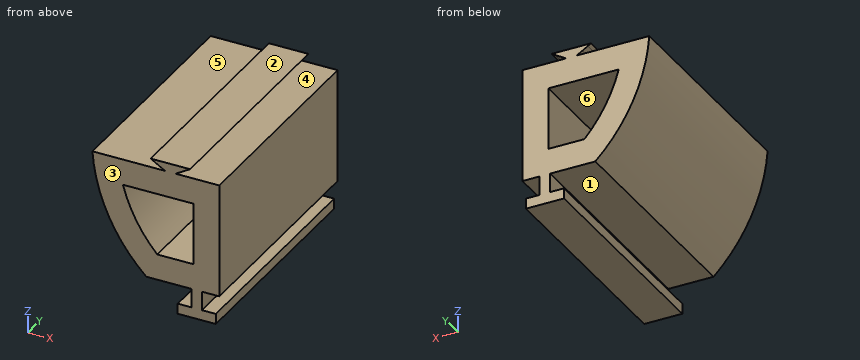
```python
from build123d import *

# Parameters (mm, degrees)
SKETCH1_W           = 0.6
SKETCH1_H           = 0.2
BOSS_EXTRUDE1_DEPTH = 13
CUT_EXTRUDE1_DEPTH  = 14


with BuildPart() as part:
    # Sketch1 → Boss-Extrude1 (new body)
    with BuildSketch(Plane(origin=(0, 0, 0), x_dir=(1, 0, 0), z_dir=(0, 1, 0))):
        with BuildLine():
            Line((-2.7, 0.7), (-2.7, 7.3))
            Line((-2.7, 7.3), (-3.7, 7.3))
            Line((-3.7, 7.3), (-4.3, 7.3))
            Line((-4.3, 7.3), (-6.907423543, 7.3))
            ThreePointArc((-6.907423543, 7.3), (-9.08690024, 4.293104241), (-10.025592252, 0.7))
            Line((-10.025592252, 0.7), (-6.025, 0.7))
            Line((-6.025, 0.7), (-5.830634937, 0.7))
            Line((-5.830634937, 0.7), (-5.219365063, 0.7))
            Line((-5.219365063, 0.7), (-5.025, 0.7))
            Line((-5.025, 0.7), (-2.7, 0.7))
        make_face()
        Polygon((-5.076449576, 0.614250707), (-5.219365063, 0.7), (-5.830634937, 0.7), (-5.973550424, 0.614250707), (-6.16396827, 0.5), (-4.88603173, 0.5), align=None)
        Polygon((-4.576449576, 0.314250707), (-4.88603173, 0.5), (-6.16396827, 0.5), (-6.473550424, 0.314250707), (-6.66396827, 0.2), (-4.38603173, 0.2), align=None)
        with Locations((-4, 7.4)):
            Rectangle(SKETCH1_W, SKETCH1_H)
        with BuildLine():
            Line((-4.3, 7.5), (-3.7, 7.5))
            Line((-3.7, 7.5), (-3.7, 8.4))
            Line((-3.7, 8.4), (-2.9, 8.4))
            Line((-2.9, 8.4), (-2.9, 9))
            Line((-2.9, 9), (-4.472415455, 9))
            ThreePointArc((-4.472415455, 9), (-4.789229045, 8.835484432), (-5.1, 8.659821014))
            Line((-5.1, 8.659821014), (-5.1, 8.4))
            Line((-5.1, 8.4), (-4.3, 8.4))
            Line((-4.3, 8.4), (-4.3, 7.5))
        make_face()
        with BuildLine():
            Line((-5.1, 8.891147283), (-5.1, 8.659821014))
            ThreePointArc((-5.1, 8.659821014), (-4.789229045, 8.835484432), (-4.472415455, 9))
            Line((-4.472415455, 9), (-4.905354218, 9))
            ThreePointArc((-4.905354218, 9), (-5.002973164, 8.946103035), (-5.1, 8.891147283))
        make_face()
        with BuildLine():
            Line((-5.1, 9), (-5.1, 8.891147283))
            ThreePointArc((-5.1, 8.891147283), (-5.002973164, 8.946103035), (-4.905354218, 9))
            Line((-4.905354218, 9), (-5.1, 9))
        make_face()
    extrude(amount=BOSS_EXTRUDE1_DEPTH)

    # Sketch2 → Cut-Extrude1 (cut, through all)
    with BuildSketch(Plane(origin=(0, 13, 0), x_dir=(1, 0, 0), z_dir=(0, 1, 0))):
        with BuildLine():
            Line((-4.2, 5.8), (-6.281918497, 5.8))
            ThreePointArc((-6.281918497, 5.8), (-7.491475696, 4.120714974), (-8.262112321, 2.2))
            Line((-8.262112321, 2.2), (-4.2, 2.2))
            Line((-4.2, 2.2), (-4.2, 5.8))
        make_face()
    extrude(amount=-CUT_EXTRUDE1_DEPTH, mode=Mode.SUBTRACT)


solid = part.part
```
The model under review builds one solid part; all positions refer to its coordinate system, in mm. Face numbers are marked on the shaded views. A direction names the side the tool comes from. Round coordinates to 2 decimals unless told otherwise and drop trailing zeros. Loops run counter-clockwise (first coordinate to the right, second up) from the corner with the lowest first, then second, coordinate; pieces in that order, holes last. Notation, with made-up numbers: (-34.5, 71) -> (15.5, 71) arc R23 cw to (15.5, 88) -> close; hole circle Ø2 at (83, 80). An arc over 180 degrees is marked (long way). Answer in a Markdown table with one row per item.
1) Tool access review of the marked faces 4, 5 and 6: name each direction out of +Z, -Z, +X, -X, +Y, -Y from which nothing blocks a thin tool from reaching the whole face with its end or side.
Taken from the geometry:
| item | result |
|---|---|
| face 4 | +X, +Y, -Y |
| face 5 | -X, +Y, -Y |
| face 6 | +Y, -Y |
2) Consider section A-A, the plane x = -5.5. Write out the cut boundary in (y, z).
Taken from the geometry:
| item | result |
|---|---|
| outline | (0, -7.3) -> (13, -7.3) -> (13, -5.8) -> (0, -5.8) -> close; (0, -2.2) -> (13, -2.2) -> (13, -0.2) -> (0, -0.2) -> close |
3) Consider section D-D, the plane z = -8. Write out the cut boundary in (x, y).
Taken from the geometry:
| item | result |
|---|---|
| outline | (-4.3, 0) -> (-3.7, 0) -> (-3.7, 13) -> (-4.3, 13) -> close |
4) For pin 1 Ø0.5 at (y, z) = (6.5, -8) entering from -X; pin 2 Ø3 at (y, z) = (5, -4) entering from -X; pin 3 Ø2 at (x, y) = (-8, 8.5) entering from +Z, all flat-tipped, find the tip position at first contact; note any pin that passes through.
Taken from the geometry:
| item | result |
|---|---|
| pin 1 | stops at x = -4.3 |
| pin 2 | stops at x = -9.73 |
| pin 3 | stops at z = -0.7 |
5) Wall thickness on line 1 along Z through (x, y) = (-5.75, 8); line 2 along Z through (x, y) = (-4.75, 8.5); line 3 along Z through (x, y) = (-3, 5.5): over which ranges is each line inside the solid? List them lowest first.
Taken from the geometry:
| item | result |
|---|---|
| line 1 | z = -7.3 to -5.8, -2.2 to -0.2 |
| line 2 | z = -9 to -8.4, -7.3 to -5.8, -2.2 to -0.7, -0.42 to -0.2 |
| line 3 | z = -9 to -8.4, -7.3 to -0.7 |
6) Consider section C-C, the plane y = 5.75. Write out the cut boundary in (x, z), plus the area to 3 significant figures.
Taken from the geometry:
| item | result |
|---|---|
| outline | (-10.03, -0.7) arc R10.05 ccw to (-6.91, -7.3) -> (-4.3, -7.3) -> (-4.3, -8.4) -> (-5.1, -8.4) -> (-5.1, -9) -> (-2.9, -9) -> (-2.9, -8.4) -> (-3.7, -8.4) -> (-3.7, -7.3) -> (-2.7, -7.3) -> (-2.7, -0.7) -> (-5.22, -0.7) -> (-4.39, -0.2) -> (-6.66, -0.2) -> (-5.83, -0.7) -> close; hole (-8.26, -2.2) arc R8.55 ccw to (-6.28, -5.8) -> (-4.2, -5.8) -> (-4.2, -2.2) -> close |
| area | 32.4 mm² |
7) Consider section B-B, the plane z = -2.5. Write out the cut boundary in (x, y).
Taken from the geometry:
| item | result |
|---|---|
| outline | (-9.73, 0) -> (-8.18, 0) -> (-8.18, 13) -> (-9.73, 13) -> close; (-4.2, 0) -> (-2.7, 0) -> (-2.7, 13) -> (-4.2, 13) -> close |
8) Draft analysis for pull direction Z (two halves, no side actions). For the marked faces 1, 2 and 3, state which applies: pulls with the +Z half, pulls with the -Z half, needs draft (parallel to the pull), parting line crosses it, or undercut.
Taken from the geometry:
| item | result |
|---|---|
| face 1 | undercut |
| face 2 | pulls with the +Z half |
| face 3 | needs draft |
